Part model, mm, in its own coordinate system. A direction names the side the tool comes from. Give positions to 0.01 mm unless a question says otherwise; leave off trailing zeros. Write each loop counter-clockwise with the first axis right and the second up, starting at its lowest first coordinate (ties: lowest second). Pieces come first, ordered by that corner, then holes.
Autodesk Inventor part; units mm, degrees
ref_plane "YZ Plane" through (0, 0, 0) normal (1, 0, 0) x (0, 1, 0)
ref_plane "XZ Plane" through (0, 0, 0) normal (0, 1, 0) x (-1, 0, 0)
ref_plane "XY Plane" through (0, 0, 0) normal (0, 0, 1) x (1, 0, 0)
sketch "Sketch1" plane through (0, 0, 0) normal (0, 0, 1) x (1, 0, 0)
  line L0 (0, 0) -> (25, 0)
  line L1 (25, 0) -> (25, 2)
  line L2 (25, 2) -> (4, 2)
  line L3 (4, 2) -> (4, 10)
  line L4 (4, 10) -> (25, 10)
  line L5 (25, 10) -> (25, 23)
  line L6 (25, 23) -> (0, 23)
  line L7 (0, 23) -> (0, 0)
  dimension "d0" = 25
  dimension "d1" = 2
  dimension "d2" = 8
  dimension "d5" = 13
extrude "Extrusion1" add sketch "Sketch1" along normal blind 23
sketch "Sketch2" plane through (0, 23, 0) normal (0, 1, 0) x (1, 0, 0)
  line L0 (0, 0) -> (25, 0)
  line L1 (25, 0) -> (25, -23)
  circle A0 centre (12.5, -11.5) radius 3
  dimension "d8" = 6
extrude "Extrusion2" cut sketch "Sketch2" against normal through all
properties part number "Eleveur support moteur"
1) Mould opens along Y. For faces 1 (the flat face through (17, 10, 11)), 2 (the cylindrical face through (10.1, 1, 13.3)), 3 (the flat face through (10, 23, 9)) say: +Y half, -Y half, draft (parallel to the pull), parting line (faces both ways), or undercut.
Check result:
face 1: undercut
face 2: draft
face 3: +Y half
2) Drill centre lines: L1, parallel to Y at x = 10.75, z = 18.5; L2, parallel to Z at x = 12.5, y = 0.7; L3, parallel to X at y = 1.55, z = 11.5. Where is each one in solid material? Low to high.
Check result:
L1: y = 0 to 2, 10 to 23
L2: z = 0 to 8.5, 14.5 to 23
L3: x = 0 to 9.5, 15.5 to 25
3) Flat gauge pins, fed straight in: P1, Ø5, axis at x = 12.5, z = 11.5, coming from the -Y side; P2, Ø4, axis at x = 13, z = 19.5, coming from the -Y side; P3, Ø2.5, axis at y = 8, z = 6.5, coming from the +X side. Where does each tip first touch, or does it go through?
Check result:
P1: passes through
P2: stops at y = 0
P3: stops at x = 4
4) Saw through at D-D (x = 6.75). Write the cut outline in (y, z), and give its area (3 significant figures).
Check result:
outline: (0, 0) - (2, 0) - (2, 23) - (0, 23) - close; (10, 0) - (23, 0) - (23, 23) - (10, 23) - close
area: 345 mm2
5) 3-axis set-ups, long thin cutter, end or side, ignore diameter. For faces 4 (the flat face through (12, 14, 23)), 5 (the flat face through (4, 6, 11)): which of +Z, -Z, +X, -X, +Y, -Y reach the whole face in a straight line?
Check result:
face 4: +Z, +X, -X, +Y, -Y
face 5: +Z, -Z, +X
6) Saw through at B-B (z = 11.5). Write the cut outline in (x, y), and give its area (3 significant figures).
Check result:
outline: (0, 0) - (9.5, 0) - (9.5, 2) - (4, 2) - (4, 10) - (9.5, 10) - (9.5, 23) - (0, 23) - close; (15.5, 0) - (25, 0) - (25, 2) - (15.5, 2) - close; (15.5, 10) - (25, 10) - (25, 23) - (15.5, 23) - close
area: 317 mm2
7) Saw through at C-C (y = 18.5). Write the cut outline in (x, z).
Check result:
outline: (0, 0) - (25, 0) - (25, 23) - (0, 23) - close; hole circle Ø6 at (12.5, 11.5)
8) Saw through at A-A (x = 12.5). Write the cut outline in (y, z).
Check result:
outline: (0, 0) - (2, 0) - (2, 8.5) - (0, 8.5) - close; (0, 14.5) - (2, 14.5) - (2, 23) - (0, 23) - close; (10, 0) - (23, 0) - (23, 8.5) - (10, 8.5) - close; (10, 14.5) - (23, 14.5) - (23, 23) - (10, 23) - close
